For this review, take the finished solid that the model builds, in its own axes (mm). A direction names the side the tool comes from. Coordinates: 2 decimals unless noted, no trailing zeros. Loops run counter-clockwise (first coordinate to the right, second up) from the corner with the lowest first, then second, coordinate; pieces in that order, holes last.
1. Clearance check with flat-ended pins moving along their axes: P1, Ø3, axis at x = 55.5, z = -16.5, coming from the +Y side; P2, Ø12, axis at x = -1, z = 8.5, coming from the +Y side. State where each tip first meets the part, or that it passes through.
2. Take a section at A-A, the plane y = 47.5. State the section outline as (x, z) points.
3. Mouldability with a two-part tool opening along Z and no side actions: class faces 5 (the face through (60, 29, -40)), 6 (the face through (6.75, 2, 14)) as pulls with the +Z half, pulls with the -Z half, needs draft (parallel to the pull), parting line crosses it, or undercut.
4. To check wall thickness, follow probe 1 along X at (y, z) = (37.5, 40); probe 2 along X at (y, z) = (0.8, 10); probe 3 along Z at (x, y) = (65, 17.5). State the ranges of each line that lie inside material, in increasing order.
5. Take a section at B-B, the plane x = 65. State the section outline as (y, z) points.
6. Take a section at C-C, the plane z = 40. State the section outline as (x, y) points.
7. Machinability: for faces 1 (the face through (60, 29, 40)), 2 (the face through (45.5, 1.5, 19.5)), 3 (the face through (63.8, 52, -41.2)), 4 (the face through (-64, 5, 33)), which of the approach directions +Z, -Z, +X, -X, +Y, -Y give a long, thin tool a straight path to every point of the face, cutting with its end or side? Answer none if there is none.
```python
from build123d import *

# Parameters (mm, degrees)
SKETCH1_W           = 140
SKETCH1_H           = 90
BOSS_EXTRUDE1_DEPTH = 2
SKETCH2_R           = 2
CUT_EXTRUDE1_DEPTH  = 84.240615087
SKETCH3_R           = 1.75
CUT_EXTRUDE2_DEPTH  = 84.240615087
SKETCH4_W           = 10
SKETCH4_H           = 10
BOSS_EXTRUDE2_DEPTH = 50
CHAMFER1_SIZE       = 5
SKETCH6_R           = 1.5
CUT_EXTRUDE3_DEPTH  = 99.127468122
CUT_EXTRUDE4_DEPTH  = 98.082439195
BOSS_EXTRUDE3_START = 1
SKETCH8_W           = 50
SKETCH8_H           = 37.5
BOSS_EXTRUDE3_DEPTH = 1
CHAMFER2_SIZE       = 1


with BuildPart() as part:
    # Sketch1 → Boss-Extrude1 (new body)
    with BuildSketch(Plane(origin=(0, 0, 0), x_dir=(1, 0, 0), z_dir=(0, 1, 0))):
        Rectangle(SKETCH1_W, SKETCH1_H)
    extrude(amount=BOSS_EXTRUDE1_DEPTH)

    # Sketch2 → Cut-Extrude1 (cut, through all)
    with BuildSketch(Plane(origin=(0, 2, 0), x_dir=(1, 0, 0), z_dir=(0, 1, 0))):
        with Locations(Location((-35, -10, 0), (0, 0, 270))):
            Circle(SKETCH2_R)
        with Locations(Location((-35, 2.5, 0), (0, 0, 270))):
            Circle(SKETCH2_R)
        with Locations(Location((-11, 11.5, 0), (0, 0, 270))):
            Circle(SKETCH2_R)
    extrude(amount=-CUT_EXTRUDE1_DEPTH, mode=Mode.SUBTRACT)

    # Sketch3 → Cut-Extrude2 (cut, through all)
    with BuildSketch(Plane(origin=(0, 2, 0), x_dir=(1, 0, 0), z_dir=(0, 1, 0))):
        with Locations(Location((45.5, 6.25, 0), (0, 0, 270))):
            Circle(SKETCH3_R)
        with Locations(Location((45.5, -13.75, 0), (0, 0, 270))):
            Circle(SKETCH3_R)
        with Locations(Location((5, 6.25, 0), (0, 0, 270))):
            Circle(SKETCH3_R)
        with Locations(Location((5, -13.75, 0), (0, 0, 270))):
            Circle(SKETCH3_R)
    extrude(amount=-CUT_EXTRUDE2_DEPTH, mode=Mode.SUBTRACT)

    # Sketch4 → Boss-Extrude2 (add)
    with BuildSketch(Plane(origin=(0, 2, 0), x_dir=(1, 0, 0), z_dir=(0, 1, 0))):
        with Locations((-65, 40)):
            Rectangle(SKETCH4_W, SKETCH4_H)
        with Locations((65, 40)):
            Rectangle(SKETCH4_W, SKETCH4_H)
        with Locations((65, -40)):
            Rectangle(SKETCH4_W, SKETCH4_H)
        with Locations((-65, -40)):
            Rectangle(SKETCH4_W, SKETCH4_H)
    extrude(amount=BOSS_EXTRUDE2_DEPTH)

    # Chamfer1
    chamfer1_edges = [part.edges().sort_by_distance(p)[0] for p in [
        (-65, 2, -35),
        (-60, 2, -40),
        (60, 2, -40),
        (65, 2, -35),
        (65, 2, 35),
        (60, 2, 40),
        (-60, 2, 40),
        (-65, 2, 35),
    ]]
    chamfer(chamfer1_edges, length=CHAMFER1_SIZE)

    # Sketch6 → Cut-Extrude3 (cut, through all)
    with BuildSketch(Plane(origin=(0, 52, 0), x_dir=(1, 0, 0), z_dir=(0, 1, 0))):
        with Locations(Location((-65, 40, 0), (0, 0, 270))):
            Circle(SKETCH6_R)
        with Locations(Location((65, 40, 0), (0, 0, 270))):
            Circle(SKETCH6_R)
        with Locations(Location((65, -40, 0), (0, 0, 270))):
            Circle(SKETCH6_R)
        with Locations(Location((-65, -40, 0), (0, 0, 270))):
            Circle(SKETCH6_R)
    extrude(amount=-CUT_EXTRUDE3_DEPTH, mode=Mode.SUBTRACT)

    # Sketch7 → Cut-Extrude4 (cut, through all)
    with BuildSketch(Plane(origin=(0, 2, 0), x_dir=(1, 0, 0), z_dir=(0, 1, 0))):
        with BuildLine():
            Line((6.75, 10.25), (6.75, 2.25))
            ThreePointArc((6.75, 2.25), (5, 0.5), (3.25, 2.25))
            Line((3.25, 2.25), (3.25, 10.25))
            ThreePointArc((3.25, 10.25), (5, 12), (6.75, 10.25))
        make_face()
        with BuildLine():
            Line((47.25, 10.25), (47.25, 2.25))
            ThreePointArc((47.25, 2.25), (45.5, 0.5), (43.75, 2.25))
            Line((43.75, 2.25), (43.75, 10.25))
            ThreePointArc((43.75, 10.25), (45.5, 12), (47.25, 10.25))
        make_face()
        with BuildLine():
            Line((6.75, -9.75), (6.75, -17.75))
            ThreePointArc((6.75, -17.75), (5, -19.5), (3.25, -17.75))
            Line((3.25, -17.75), (3.25, -9.75))
            ThreePointArc((3.25, -9.75), (5, -8), (6.75, -9.75))
        make_face()
        with BuildLine():
            Line((43.75, -17.75), (43.75, -9.75))
            ThreePointArc((43.75, -9.75), (45.5, -8), (47.25, -9.75))
            Line((47.25, -9.75), (47.25, -17.75))
            ThreePointArc((47.25, -17.75), (45.5, -19.5), (43.75, -17.75))
        make_face()
    extrude(amount=-CUT_EXTRUDE4_DEPTH, mode=Mode.SUBTRACT)

    # Sketch8 → Boss-Extrude3 (add)
    with BuildSketch(Plane(origin=(0, 2, 0), x_dir=(1, 0, 0), z_dir=(0, 1, 0)).offset(BOSS_EXTRUDE3_START)):
        with Locations((25.25, -3.75)):
            Rectangle(SKETCH8_W, SKETCH8_H)
        with BuildLine():
            Line((47.25, 2.25), (47.25, 10.25))
            ThreePointArc((47.25, 10.25), (45.5, 12), (43.75, 10.25))
            Line((43.75, 10.25), (43.75, 2.25))
            ThreePointArc((43.75, 2.25), (45.5, 0.5), (47.25, 2.25))
        make_face(mode=Mode.SUBTRACT)
        with BuildLine():
            Line((3.25, 10.25), (3.25, 2.25))
            ThreePointArc((3.25, 2.25), (5, 0.5), (6.75, 2.25))
            Line((6.75, 2.25), (6.75, 10.25))
            ThreePointArc((6.75, 10.25), (5, 12), (3.25, 10.25))
        make_face(mode=Mode.SUBTRACT)
        with BuildLine():
            Line((47.25, -17.75), (47.25, -9.75))
            ThreePointArc((47.25, -9.75), (45.5, -8), (43.75, -9.75))
            Line((43.75, -9.75), (43.75, -17.75))
            ThreePointArc((43.75, -17.75), (45.5, -19.5), (47.25, -17.75))
        make_face(mode=Mode.SUBTRACT)
        with BuildLine():
            Line((3.25, -9.75), (3.25, -17.75))
            ThreePointArc((3.25, -17.75), (5, -19.5), (6.75, -17.75))
            Line((6.75, -17.75), (6.75, -9.75))
            ThreePointArc((6.75, -9.75), (5, -8), (3.25, -9.75))
        make_face(mode=Mode.SUBTRACT)
    extrude(amount=-BOSS_EXTRUDE3_DEPTH)

    # Chamfer2
    chamfer2_edges = [part.edges().sort_by_distance(p)[0] for p in [
        (50.25, 2, 3.75),
        (25.25, 2, -15),
        (0.25, 2, 3.75),
        (25.25, 2, 22.5),
    ]]
    chamfer(chamfer2_edges, length=CHAMFER2_SIZE - 0.0001)  # a hair under: the kernel refuses the full size


solid = part.part
```
Results list:
1. P1: stops at y = 2
1. P2: stops at y = 3
2. outline: (-70, -45) - (-60, -45) - (-60, -35) - (-70, -35) - close; (-70, 35) - (-60, 35) - (-60, 45) - (-70, 45) - close; (60, -45) - (70, -45) - (70, -35) - (60, -35) - close; (60, 35) - (70, 35) - (70, 45) - (60, 45) - close; hole circle Ø3 at (-65, -40); hole circle Ø3 at (-65, 40); hole circle Ø3 at (65, -40); hole circle Ø3 at (65, 40)
3. face 5: needs draft
3. face 6: undercut
4. probe 1: x = -70 to -66.5, -63.5 to -60, 60 to 63.5, 66.5 to 70
4. probe 2: x = -70 to -37, -33 to 3.25, 6.75 to 43.75, 47.25 to 70
4. probe 3: z = -45 to -41.5, -38.5 to -35, 35 to 38.5, 41.5 to 45
5. outline: (0, -45) - (52, -45) - (52, -41.5) - (0, -41.5) - close; (0, -38.5) - (52, -38.5) - (52, -35) - (7, -35) - (2, -30) - (2, 30) - (7, 35) - (52, 35) - (52, 38.5) - (0, 38.5) - close; (0, 41.5) - (52, 41.5) - (52, 45) - (0, 45) - close
6. outline: (-70, 0) - (-66.5, 0) - (-66.5, 52) - (-70, 52) - close; (-63.5, 0) - (63.5, 0) - (63.5, 52) - (60, 52) - (60, 7) - (55, 2) - (-55, 2) - (-60, 7) - (-60, 52) - (-63.5, 52) - close; (66.5, 0) - (70, 0) - (70, 52) - (66.5, 52) - close
7. face 1: +Z, -Z, +Y
7. face 2: +Y, -Y
7. face 3: +Z, -Z, +X, -X, +Y
7. face 4: +X, -X, +Y
